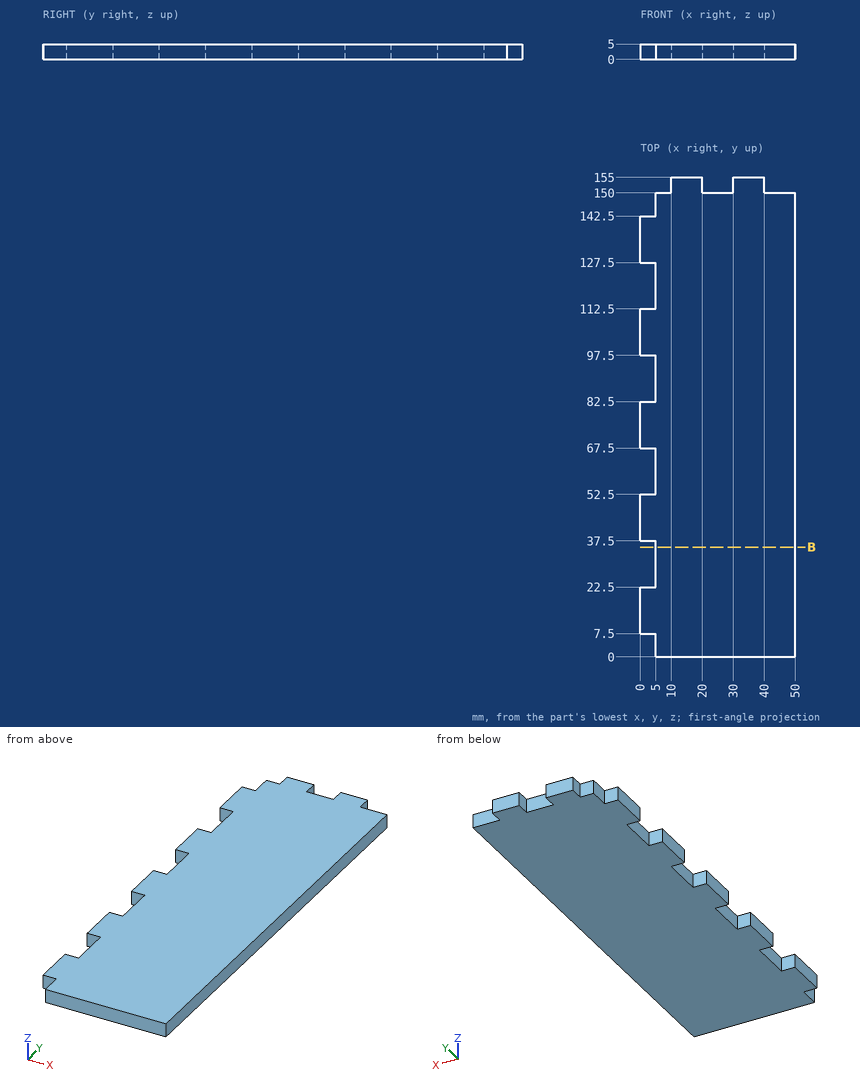
Study the drawing (mm; zero at the part's minimum x, y, z) and answer. Round coordinates to 2 decimals unless told otherwise and drop trailing zeros. Write each loop counter-clockwise with the first axis right and the second up, starting at its lowest first coordinate (ties: lowest second). Pieces come first, ordered by that corner, then holes. Notation, with made-up numbers: (81.5, -25) -> (109.5, -25) arc R29 cw to (109.5, 6) -> close; hole circle Ø2 at (9, 66). An arc over 180 degrees is marked (long way). Write item = value, one per line.
1) Section B-B on y = 35.5 is taken. Write down the section's boundary in (x, z).
Check values:
outline = (5, 0) -> (50, 0) -> (50, 5) -> (5, 5) -> close
2) Straight lines are drawn through the part: line 1 along Y through (x, z) = (4, 3.7); line 2 along Y through (x, z) = (46, 3); line 3 along X through (y, z) = (85, 3.05). For each, find the intervals that lie inside material, in ascending order. Write a range as [from, to].
Check values:
line_1 = [7.5, 22.5], [37.5, 52.5], [67.5, 82.5], [97.5, 112.5], [127.5, 142.5]
line_2 = [0, 150]
line_3 = [5, 50]
3) Given pin 1 (1.5 mm diameter, centred on x = 6.5, z = 1.5, fed in from +Y); pin 2 (1.5 mm diameter, centred on x = 3.5, z = 3, fed in from -Y); pin 3 (1.5 mm diameter, centred on y = 62, z = 3, fed in from -X), each flat-ended and moving along its own axis, determine where each tip first touches the part or whether it passes through.
Check values:
pin_1 = 150
pin_2 = 7.5
pin_3 = 5
